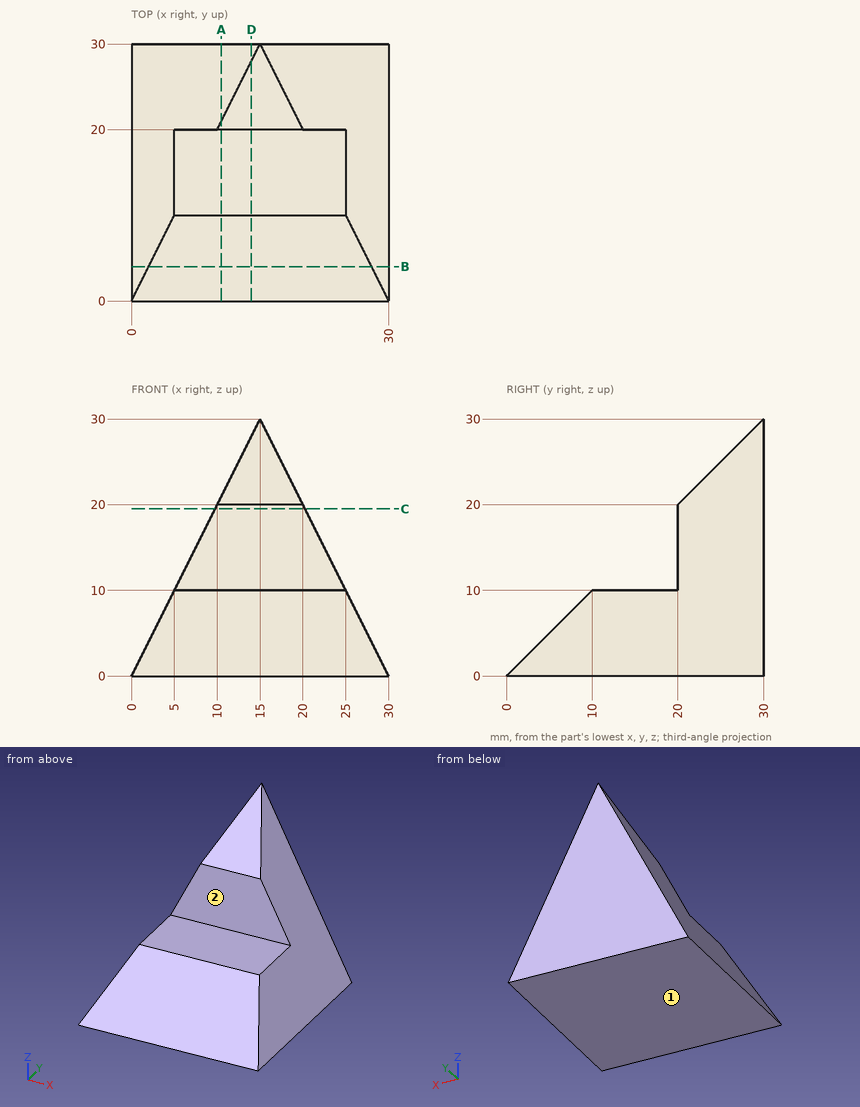
Drawing for the job (mm, zero at the part's lowest x, y, z). A direction names the side the tool comes from. Coordinates: 2 decimals unless noted, no trailing zeros. Order: outer loops, then holes, each group sorted by start corner. A loop starts at its lowest first (then second) coordinate and runs counter-clockwise, first axis right, second up. Notation, with made-up numbers: (-29.5, 55) -> (24.5, 55) arc R22 ccw to (24.5, 63) -> close; hole circle Ø1 at (5.25, 17.25). An arc over 180 degrees is marked (long way). Answer in a Markdown table with one row per item.
1) Flat gauge pins, fed straight in: P1, Ø10, axis at x = 16, y = 24, coming from the +Z side; P2, Ø5, axis at x = 15, y = 16.5, coming from the +Z side; P3, Ø12, axis at x = 16, z = 7, coming from the -Y side; P4, Ø6, axis at x = 25.5, y = 12.5, coming from the -Z side. Where does each tip first touch, or does it go through?
Check values:
| item | result |
|---|---|
| P1 | z = 28.98 |
| P2 | z = 10 |
| P3 | y = 1 |
| P4 | z = 0 |
2) Band-saw the part on D-D (x = 14). List the corners of the cut face in (y, z), and give its area (3 significant figures).
Check values:
| item | result |
|---|---|
| outline | (0, 0) -> (30, 0) -> (30, 28) -> (28, 28) -> (20, 20) -> (20, 10) -> (10, 10) -> close |
| area | 398 mm2 |
3) Which spindle directions (+Z, -Z, +X, -X, +Y, -Y) get a long thin tool onto all of the face, cutting with end or side? Do the marked faces 1 and 2. Say none if no direction does.
Check values:
| item | result |
|---|---|
| face 1 | -Z, +X, -X, +Y, -Y |
| face 2 | +Z, +X, -X, -Y |
4) Band-saw the part on A-A (x = 10.5). List the corners of the cut face in (y, z), and give its area (4 significant figures).
Check values:
| item | result |
|---|---|
| outline | (0, 0) -> (30, 0) -> (30, 21) -> (21, 21) -> (20, 20) -> (20, 10) -> (10, 10) -> close |
| area | 359.5 mm2 |
5) Band-saw the part on B-B (y = 4). List the corners of the cut face in (x, z), and give its area (3 significant figures).
Check values:
| item | result |
|---|---|
| outline | (0, 0) -> (30, 0) -> (28, 4) -> (2, 4) -> close |
| area | 112 mm2 |
6) Band-saw the part on C-C (z = 19.5). List the corners of the cut face in (x, y).
Check values:
| item | result |
|---|---|
| outline | (9.75, 20) -> (20.25, 20) -> (20.25, 30) -> (9.75, 30) -> close |
7) Drill centre lines: line 1 (Y direction, x = 7.75, z = 11.5); line 2 (Z direction, x = 17, y = 15); line 3 (X direction, y = 20.5, z = 17). Where is each one in solid material? Low to high.
Check values:
| item | result |
|---|---|
| line 1 | 20 to 30 |
| line 2 | 0 to 10 |
| line 3 | 8.5 to 21.5 |
